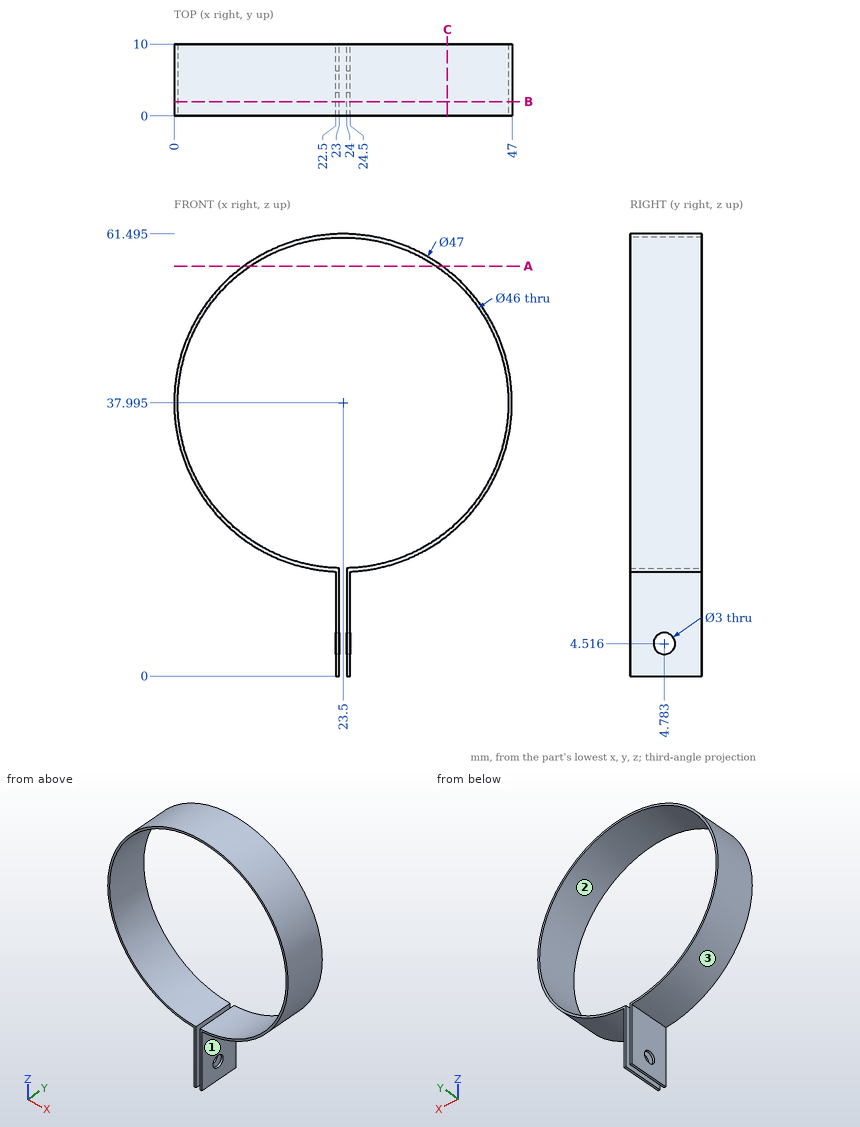
Job drawing, mm, ordinate dimensions from the low corner. One solid piece. Coordinates: 2 decimals unless noted, no trailing zeros. Write each loop counter-clockwise with the first axis right and the second up, starting at its lowest first coordinate (ties: lowest second). Pieces come first, ordered by that corner, then holes. Notation, with made-up numbers: (87.25, -37.75) -> (111.25, -37.75) arc R25 cw to (111.25, -14.75) -> close; hole circle Ø9 at (70.25, 26). An arc over 180 degrees is marked (long way). Use CSV: the item, a comma, the result in double quotes. Start each with the question number.
Item 1: Band-saw the part on A-A, the plane z = 57. Write the cut outline in (x, y).
Item 2: Two-plate mould, pull along X, no slides. Class the marked faces 1, 2 and 3: +X half, -X half, draft (parallel to the pull), parting line (faces both ways), or undercut.
Item 3: Drop flat-ended pins along their axis: P1, Ø3, axis at y = 6.5, z = 9, coming from the +X side; P2, Ø3.5, axis at y = 4.78, z = 4.52, coming from the -X side; P3, Ø2, axis at x = 28, y = 9, coming from the -Z side; P4, Ø10, axis at x = 10, z = 45, coming from the +Y side. Give the stop position or say it passes through.
Item 4: Band-saw the part on B-B, the plane y = 2. Write the cut outline in (x, z) (1 decimal).
Item 5: Wall check: probe 1 along X at (y, z) = (9.75, 37.5) (1 decimal); probe 2 along X at (y, z) = (1.25, 6); probe 3 along Z at (x, y) = (20, 4.25). Give the ranges that are in metal, low to high.
Item 6: Band-saw the part on C-C, the plane x = 38. Write the cut outline in (y, z), plus the area to 3 significant figures.
Response values:
1,outline,"(9.68, 0) -> (10.55, 0) -> (10.55, 10) -> (9.68, 10) -> close; (36.45, 0) -> (37.32, 0) -> (37.32, 10) -> (36.45, 10) -> close"
2,face 1,"+X half"
2,face 2,"undercut"
2,face 3,"parting line"
3,P1,"stops at x = 24.5"
3,P2,"stops at x = 22.5"
3,P3,"stops at z = 14.76"
3,P4,"passes through"
4,outline,"(22.5, 0) -> (23, 0) -> (23, 15) arc R23 cw (long way) to (24, 15) -> (24, 0) -> (24.5, 0) -> (24.5, 14.5) arc R23.5 ccw (long way) to (22.5, 14.5) -> close"
5,probe 1,"x = 0 to 0.5, 46.5 to 47"
5,probe 2,"x = 22.5 to 23, 24 to 24.5"
5,probe 3,"z = 14.76 to 15.26, 60.73 to 61.23"
6,outline,"(0, 19.5) -> (10, 19.5) -> (10, 20.14) -> (0, 20.14) -> close; (0, 55.85) -> (10, 55.85) -> (10, 56.49) -> (0, 56.49) -> close"
6,area,"12.8 mm2"
